from build123d import *

# Parameters (mm, degrees)
SKETCH2_W               = 18.5
SKETCH2_H               = 25.41
BOSS_EXTRUDE1_DEPTH     = 9
CUT_EXTRUDE1_DEPTH      = 25.41
CUT_EXTRUDE3_DEPTH      = 33.694312961
CUT_EXTRUDE3_DEPTH_BACK = 25.41
SKETCH10_R              = 1.22
CUT_EXTRUDE4_DEPTH      = 33.694312961


with BuildPart() as part:
    # Sketch2 → Boss-Extrude1 (new body)
    with BuildSketch(Plane(origin=(0, 0, 0), x_dir=(1, 0, 0), z_dir=(0, 1, 0))):
        with Locations((9.25, 12.705)):
            Rectangle(SKETCH2_W, SKETCH2_H)
    extrude(amount=BOSS_EXTRUDE1_DEPTH)

    # Sketch6 → Cut-Extrude1 (cut)
    with BuildSketch(Plane.XY):
        with BuildLine():
            Line((2.9, 9), (15.6, 9))
            ThreePointArc((15.6, 9), (9.25, 2.65), (2.9, 9))
        make_face()
    extrude(amount=-CUT_EXTRUDE1_DEPTH, mode=Mode.SUBTRACT)

    # Sketch14 → Cut-Extrude3 (cut, two sides: drawn at the far end of the back side and taken through both)
    with BuildSketch(Plane(origin=(0, 0, -25.41), x_dir=(-1, 0, 0), z_dir=(0, 0, -1)).offset(-CUT_EXTRUDE3_DEPTH_BACK)):
        Polygon((0, 60.146081223), (0, 9), (0, 7.5), (-3.246658661, 7.5), (-2.9, 9), (8.616604878, 58.832614185), (24.031387378, 159.956651774), (15.4147825, 161.270118812), align=None)
    extrude(amount=CUT_EXTRUDE3_DEPTH + CUT_EXTRUDE3_DEPTH_BACK, mode=Mode.SUBTRACT)


with BuildPart() as cut_extrude3_kept_piece:
    # of the separate pieces the step leaves, the one the design keeps (cut_extrude3_pieces_kept)
    add(part.part.solids().sort_by_distance((0, 0, 0))[0])

    # Sketch10 → Cut-Extrude4 (cut, through all)
    with BuildSketch(Plane(origin=(0, 9, 0), x_dir=(1, 0, 0), z_dir=(0, 1, 0))):
        with Locations(Location((17.05, 20.41, 0), (0, 0, 270))):
            Circle(SKETCH10_R)
        with Locations(Location((17.05, 5, 0), (0, 0, 270))):
            Circle(SKETCH10_R)
    extrude(amount=-CUT_EXTRUDE4_DEPTH, mode=Mode.SUBTRACT)


solid = cut_extrude3_kept_piece.part
Check sheet for the modelled part. Datum: model origin and axes. Units: mm. A direction names the side the tool comes from. Round coordinates to 2 decimals unless told otherwise and drop trailing zeros. Order: outer loops, then holes, each group sorted by start corner. A loop starts at its lowest first (then second) coordinate and runs counter-clockwise, first axis right, second up. Notation, with made-up numbers: M 86.25,87 L 132.25,87 A19 ccw 132.25,101 Z; hole C -9,-39 d6. An arc over 180 degrees is marked long. One line per item, written item: value. Start each with the question number.
1. Section check B-B on x = 17.05. Enter the section's corners in (y, z), and give its area (3 significant figures).
2. Access from +Z, -Z, +X, -X, +Y, -Y to the whole of each face (thin tool, end or side, straight path). Record for faces 4 (the flat face through (2, 7.5, -13)), 5 (the flat face through (9, 2, -25.41)).
3. Section check C-C on y = 1.75. Enter the section's corners in (x, z), and give its area (3 significant figures).
4. Gauge pin test, flat ends, axial feed: P1, Ø3.5, axis at x = 1.5, z = -17, coming from the +Y side; P2, Ø1.5, axis at x = 6.5, z = -7.5, coming from the +Y side. Record the tip position at first contact, or that the pin passes through.
5. Scan lines: line 1 along X through (y, z) = (6, -20.41); line 2 along Z through (x, y) = (17.75, 1.5); line 3 along X through (y, z) = (5.25, -20.41). Record each from-to range of solid material in increasing order.
6. Section check A-A on z = -5. Enter the section's corners in (x, y), and give its area (3 significant figures).
7. Section check D-D on x = 4. Enter the section's corners in (y, z).
8. Release check for a two-part mould opening along Z. For faces 1 (the flat face through (17, 9, -13)), 2 (the cylindrical face through (18.26, 4.56, -5.16)), 3 (the flat face through (9, 2, 0)) record: released by +Z, released by -Z, zero draft, split by the parting line, or undercut.
Results found:
1. outline: M 0,-25.41 L 9,-25.41 L 9,-21.63 L 0,-21.63 Z; M 0,-19.19 L 9,-19.19 L 9,-6.22 L 0,-6.22 Z; M 0,-3.78 L 9,-3.78 L 9,0 L 0,0 Z
1. area: 185 mm^2
2. face 4: +Z, -Z, -X, +Y
2. face 5: -Z, +X, -X, +Y, -Y
3. outline: M 0,-25.41 L 18.5,-25.41 L 18.5,0 L 0,0 Z; hole C 17.05,-20.41 d2.44; hole C 17.05,-5 d2.44
3. area: 461 mm^2
4. P1: y = 7.5
4. P2: y = 3.7
5. line 1: 0 to 3.65, 14.85 to 15.83, 18.27 to 18.5
5. line 2: -25.41 to -21.41, -19.41 to -6, -4 to 0
5. line 3: 0 to 4.13, 14.37 to 15.83, 18.27 to 18.5
6. outline: M 0,0 L 15.83,0 L 15.83,9 L 15.6,9 A6.35 cw 3.08,7.5 L 0,7.5 Z; M 18.27,0 L 18.5,0 L 18.5,9 L 18.27,9 Z
6. area: 76.8 mm^2
7. outline: M 0,-25.41 L 5.43,-25.41 L 5.43,0 L 0,0 Z
8. face 1: zero draft
8. face 2: undercut
8. face 3: released by +Z
